from build123d import *

# Parameters (mm, degrees)
F0_R     = 7.5
F1_DEPTH = 24
F2_R     = 5


with BuildPart() as f1:
    # F0 (on Top) → F1 (new body, symmetric)
    with BuildSketch(Plane.XY):
        with BuildLine():
            Line((-17.5, 13.5), (-26.833323, 9.012342))
            ThreePointArc((-26.833323, 9.012342), (-27.822911, -8.465614), (-12.5, 0))
            Line((-12.5, 0), (-11.5, 0))
            Line((-11.5, 0), (-11.5, 11))
            Line((-11.5, 11), (11.5, 11))
            Line((11.5, 11), (11.5, 0))
            Line((11.5, 0), (12.5, 0))
            ThreePointArc((12.5, 0), (27.822911, -8.465614), (26.833323, 9.012342))
            Line((26.833323, 9.012342), (17.5, 13.5))
            Line((17.5, 13.5), (-17.5, 13.5))
        make_face()
        with Locations((-22.5, 0)):
            Circle(F0_R, mode=Mode.SUBTRACT)
        with Locations((22.5, 0)):
            Circle(F0_R, mode=Mode.SUBTRACT)
    extrude(amount=F1_DEPTH, both=True)

    # F2
    f2_edges = [f1.edges().sort_by_distance(p)[0] for p in [
        (17.5, 13.5, 0),
        (-17.5, 13.5, 0),
    ]]
    fillet(f2_edges, radius=F2_R)


solid = f1.part
Design review of the part built by this model. Coordinates are the model's own, in mm. A direction names the side the tool comes from. Round coordinates to 2 decimals unless told otherwise and drop trailing zeros. Write each loop counter-clockwise with the first axis right and the second up, starting at its lowest first coordinate (ties: lowest second). Pieces come first, ordered by that corner, then holes. Notation, with made-up numbers: (22.25, 5) - (29.25, 5) arc R22 cw to (29.25, 40) - close; hole circle Ø3 at (84.25, 41.5). An arc over 180 degrees is marked (long way). Use a Markdown table: item, result. Add a question column.
1. We need section D-D (x = 9). State the section outline as (y, z) points.
2. Wall thickness on probe 1 along X at (y, z) = (-0.25, -10); probe 2 along X at (y, z) = (2, -18); probe 3 along X at (y, z) = (7.75, -16): over which ranges is each line inside the solid? List them lowest first.
3. Mouldability with a two-part tool opening along Y and no side actions: class faces 3 (the face through (-17.49, 13.37, -0.34)), 4 (the face through (-30, 0, 0)), 5 (the face through (15, 0, 0)), 6 (the face through (11.5, 6, 0)) as +Y half, -Y half, draft (parallel to the pull), parting line (faces both ways), or undercut.
4. For faces 1 (the face through (0, 11, 0)), 2 (the face through (-28.073, -8.303, 0.336)), list the 3-axis set-ups (+Z, -Z, +X, -X, +Y, -Y) from which the entire face can be reached by the end or side of a thin tool; tool diameter is ignored.
5. We need section B-B (y = -2.25). State the section outline as (x, z) points.
6. Clearance check with flat-ended pins moving along their axes: pin 1 (2 mm diameter, centred on y = -4.5, z = 7, fed in from -X); pin 2 (11.5 mm diameter, centred on x = 3, z = -6, fed in from -Y); pin 3 (0.8 mm diameter, centred on x = -12, z = 7, fed in from -Y). State where each tip first meets the part, or that it passes through.
7. We need section A-A (z = -12). State the section outline as (x, y) points.
8. We need section C-C (x = -22). State the section outline as (y, z) points.
Output:
| question | item | result |
|---|---|---|
| 1 | outline | (11, -24) - (13.5, -24) - (13.5, 24) - (11, 24) - close |
| 2 | probe 1 | x = -32.5 to -30, -15 to -12.5, 12.5 to 15, 30 to 32.5 |
| 2 | probe 2 | x = -32.3 to -29.73, -15.27 to -11.5, 11.5 to 15.27, 29.73 to 32.3 |
| 2 | probe 3 | x = -28.82 to -11.5, 11.5 to 28.82 |
| 3 | face 3 | +Y half |
| 3 | face 4 | undercut |
| 3 | face 5 | undercut |
| 3 | face 6 | draft |
| 4 | face 1 | +Z, -Z, -Y |
| 4 | face 2 | +Z, -Z |
| 5 | outline | (-32.24, -24) - (-29.65, -24) - (-29.65, 24) - (-32.24, 24) - close; (-15.35, -24) - (-12.76, -24) - (-12.76, 24) - (-15.35, 24) - close; (12.76, -24) - (15.35, -24) - (15.35, 24) - (12.76, 24) - close; (29.65, -24) - (32.24, -24) - (32.24, 24) - (29.65, 24) - close |
| 6 | pin 1 | stops at x = -31.87 |
| 6 | pin 2 | stops at y = 11 |
| 6 | pin 3 | stops at y = 0 |
| 7 | outline | (-26.83, 9.01) arc R10 ccw (long way) to (-12.5, 0) - (-11.5, 0) - (-11.5, 11) - (11.5, 11) - (11.5, 0) - (12.5, 0) arc R10 ccw (long way) to (26.83, 9.01) - (18.53, 13.01) arc R5 ccw to (16.36, 13.5) - (-16.36, 13.5) arc R5 ccw to (-18.53, 13.01) - close; hole circle Ø15 at (-22.5, 0); hole circle Ø15 at (22.5, 0) |
| 8 | outline | (-9.99, -24) - (-7.48, -24) - (-7.48, 24) - (-9.99, 24) - close; (7.48, -24) - (11.34, -24) - (11.34, 24) - (7.48, 24) - close |
